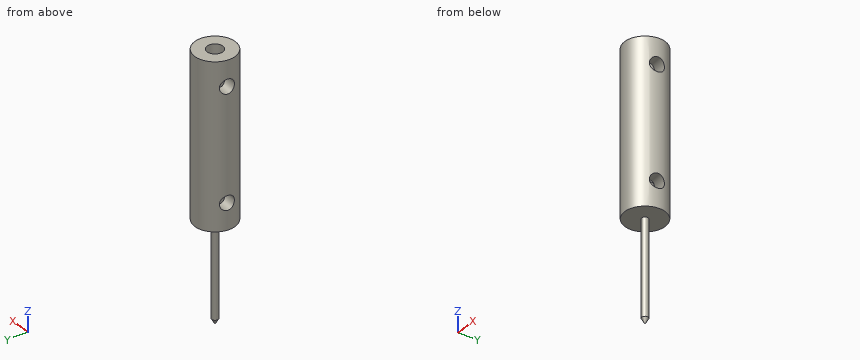
from build123d import *

# Parameters (mm, degrees)
SKETCH3_R                           = 3.2
SKETCH3_R_2                         = 0.5
BOSS_EXTRUDE2_DEPTH                 = 25.7
CUT_EXTRUDE1_DEPTH                  = 27.095401894
CUT_EXTRUDE1_DEPTH_BACK             = 25.7
SKETCH6_R                           = 1.25
TAP_DRILL_FOR_4_40_TAP1_D           = 2.2606
TAP_DRILL_FOR_4_40_TAP1_ON_FACE_2_D = 2.2606
BOSS_EXTRUDE4_START                 = 5
SKETCH3_4_R                         = 0.5
BOSS_EXTRUDE4_DEPTH                 = 20
BOSS_EXTRUDE5_START                 = -20.7
SKETCH6_2_R                         = 1.25
SKETCH6_2_R_2                       = 0.5
BOSS_EXTRUDE5_DEPTH                 = 5


with BuildPart() as part:
    # Sketch3 → Boss-Extrude2 (new body)
    with BuildSketch(Plane.XY):
        with Locations(Location((0, 0, 0), (0, 0, 180))):
            Circle(SKETCH3_R)
        Circle(SKETCH3_R_2, mode=Mode.SUBTRACT)
    extrude(amount=BOSS_EXTRUDE2_DEPTH)

    # Sketch6 → Cut-Extrude1 (cut, two sides: drawn at the far end of the back side and taken through both)
    with BuildSketch(Plane.XY.offset(25.7).offset(-CUT_EXTRUDE1_DEPTH_BACK)):
        with Locations(Location((0, 0, 0), (0, 0, 180))):
            Circle(SKETCH6_R)
    extrude(amount=CUT_EXTRUDE1_DEPTH + CUT_EXTRUDE1_DEPTH_BACK, mode=Mode.SUBTRACT)

    # Tap Drill for #4-40 Tap1 (through all)
    with Locations(Plane(origin=(3.187528357, -0.282246299, 21.7), x_dir=(0.088201968553, 0.996102611553, 0), z_dir=(0.996102611553, -0.088201968553, 0))):
        with Locations((0, 0)):
            Hole(TAP_DRILL_FOR_4_40_TAP1_D / 2)

    # Tap Drill for #4-40 Tap1 on face 2 (through all)
    with Locations(Plane(origin=(3.187528357, -0.282246299, 4.112360987), x_dir=(0.088201965627, 0.996102611812, 0), z_dir=(0.996102611812, -0.088201965627, 0))):
        with Locations((0, 0)):
            Hole(TAP_DRILL_FOR_4_40_TAP1_ON_FACE_2_D / 2)



with BuildPart() as body_2:
    # Sketch3<4> → Boss-Extrude4 (new body)
    with BuildSketch(Plane.XY.offset(BOSS_EXTRUDE4_START)):
        Circle(SKETCH3_4_R)
    extrude(amount=-BOSS_EXTRUDE4_DEPTH)

    # Sketch9 → Revolve1 (revolve)
    with BuildSketch(Plane(origin=(0, 0, 0), x_dir=(1, 0, 0), z_dir=(0, 1, 0)), mode=Mode.PRIVATE) as revolve1_sk:
        Polygon((0, 15), (-0.5, 15), (0, 15.866025404), align=None)
    revolve(revolve1_sk.sketch.rotate(Axis((0, 0, -15), (0, 0, -1)), 180), axis=Axis((0, 0, -15), (0, 0, -1)))


with BuildPart() as part_1:
    add(part.part)

    add(body_2.part)  # Boss-Extrude5 merges body 2
    # Sketch6<2> → Boss-Extrude5 (add)
    with BuildSketch(Plane.XY.offset(25.7).offset(BOSS_EXTRUDE5_START)):
        with Locations(Location((0, 0, 0), (0, 0, 208.982799993))):
            Circle(SKETCH6_2_R)
        Circle(SKETCH6_2_R_2, mode=Mode.SUBTRACT)
    extrude(amount=-BOSS_EXTRUDE5_DEPTH)


solid = part_1.part
Input: part model. Units: mm. Frame: model coordinates. Give positions to 0.01 mm unless a question says otherwise; leave off trailing zeros. Order: outer loops, then holes, each group sorted by start corner. A loop starts at its lowest first (then second) coordinate and runs counter-clockwise, first axis right, second up. Notation, with made-up numbers: M -28,52.25 L -18,52.25 A30 ccw -18,76.25 Z; hole C 21.25,79.5 d3. An arc over 180 degrees is marked long. Answer as a JSON object with one key per item and string values.
1. Cut plane C-C, the plane x = 2.5. State how many separate pieces and enclosed holes the cut face has, and give its area (3 significant figures).
Result sheet:
{"separate pieces": "1", "enclosed holes": "2", "area": "94.6 mm²"}
2. Ray query, line 1 (Z direction, x = 2.75, y = -0.25); line 2 (Y direction, x = 0, z = 20.25); line 3 (Z direction, x = 0.25, y = -2.5). Return the intervals inside material, ascending. Write a range as [from, to].
Result sheet:
{"line 1": "[0, 2.98], [5.24, 20.57], [22.83, 25.7]", "line 2": "[-3.2, -1.25], [1.25, 3.2]", "line 3": "[0, 25.7]"}
3. First-contact query: P1, Ø2, axis at x = 0, y = 0, coming from the +Z side; P2, Ø2, axis at x = 2.5, z = 13, coming from the -Y side. Flat tips, straight axial feed; report the tip coordinate or a pass-through.
Result sheet:
{"P1": "z = 5", "P2": "y = -2.83"}
4. Cut plane B-B, the plane z = -3.5. Output: boundary loops of the cut face in (x, y).
Result sheet:
{"outline": "C 0,0 d1"}
5. Cut plane D-D, the plane y = -2.5. Output: boundary loops of the cut face in (x, z), and give its area (3 significant figures).
Result sheet:
{"outline": "M -2,0 L 2,0 L 2,25.7 L -2,25.7 Z", "area": "103 mm²"}
6. Cut plane A-A, the plane z = 13.5. Output: boundary loops of the cut face in (x, y).
Result sheet:
{"outline": "C 0,0 d6.4; hole C 0,0 d2.5"}
